Geometry: final body of the model. Coordinates: model frame, mm. A direction names the side the tool comes from. Coordinates: 2 decimals unless noted, no trailing zeros. Order: outer loops, then holes, each group sorted by start corner. A loop starts at its lowest first (then second) coordinate and runs counter-clockwise, first axis right, second up. Notation, with made-up numbers: (28.5, 34.5) -> (40.5, 34.5) arc R15 ccw to (40.5, 48.5) -> close; hole circle Ø5 at (17.25, -19.75). An arc over 180 degrees is marked (long way). Use one line per item in the form item = value.
```python
from build123d import *

# Parameters (mm, degrees)
SKETCH1_R               = 7.5
BOSS_EXTRUDE1_DEPTH     = 240
SKETCH5_R               = 8
BOSS_EXTRUDE2_DEPTH     = 20
SKETCH8_R               = 5
BOSS_EXTRUDE4_DEPTH     = 8
SKETCH9_R               = 2.5
CUT_EXTRUDE3_DEPTH      = 8
CUT_EXTRUDE3_DEPTH_BACK = 8


with BuildPart() as part:
    # Sketch1 → Boss-Extrude1 (new body)
    with BuildSketch(Plane.XY):
        Circle(SKETCH1_R)
    extrude(amount=BOSS_EXTRUDE1_DEPTH)

    # Sketch5 → Boss-Extrude2 (add)
    with BuildSketch(Plane.XY.offset(240)):
        Circle(SKETCH5_R)
    extrude(amount=BOSS_EXTRUDE2_DEPTH)

    # Sketch8 → Boss-Extrude4 (add)
    with BuildSketch(Plane(origin=(0, 0, 0), x_dir=(-1, 0, 0), z_dir=(0, 0, -1))):
        Circle(SKETCH8_R)
    extrude(amount=BOSS_EXTRUDE4_DEPTH)

    # Sketch9 → Cut-Extrude3 (cut, two sides)
    with BuildSketch(Plane(origin=(0, 0, 0), x_dir=(1, 0, 0), z_dir=(0, 1, 0))) as cut_extrude3_sk:
        with Locations((0, -250.064612311)):
            Circle(SKETCH9_R)
    extrude(amount=CUT_EXTRUDE3_DEPTH, mode=Mode.SUBTRACT)
    extrude(cut_extrude3_sk.sketch, amount=-CUT_EXTRUDE3_DEPTH_BACK, mode=Mode.SUBTRACT)


solid = part.part
```
1) Section A-A, the plane x = 0. Output: boundary loops of the cut face in (y, z), and give its area (3 significant figures).
Results found:
outline = (-8, 240) -> (-7.5, 240) -> (-7.5, 0) -> (-5, 0) -> (-5, -8) -> (5, -8) -> (5, 0) -> (7.5, 0) -> (7.5, 240) -> (8, 240) -> (8, 247.56) -> (-8, 247.56) -> close; (-8, 252.56) -> (8, 252.56) -> (8, 260) -> (-8, 260) -> close
area = 3,920 mm2
2) Section C-C, the plane z = 170.5. Output: boundary loops of the cut face in (x, y).
Results found:
outline = circle Ø15 at (0, 0)
3) Pull-direction query (Z, two-part tool) for faces 3 (the cylindrical face through (-0.542, -0.112, 252.505)), 4 (the flat face through (0, 0, -8)), 5 (the cylindrical face through (1.08, -4.88, -3.94)); classes: released by +Z, released by -Z, zero draft, split by the parting line, or undercut.
Results found:
face_3 = undercut
face_4 = released by -Z
face_5 = zero draft
4) Contact query for flat-ended pins moving along their axis: P1, Ø4, axis at x = -5, z = 123.5, coming from the -Y side; P2, Ø8, axis at x = -6, z = 91.5, coming from the +Y side; P3, Ø3, axis at y = -2, z = 43.5, coming from the +X side. Output: stop coordinate, or through.
Results found:
P1 = -6.87
P2 = 7.23
P3 = 7.48
5) Section B-B, the plane y = 0. Output: boundary loops of the cut face in (x, z).
Results found:
outline = (-8, 240) -> (-7.5, 240) -> (-7.5, 0) -> (-5, 0) -> (-5, -8) -> (5, -8) -> (5, 0) -> (7.5, 0) -> (7.5, 240) -> (8, 240) -> (8, 260) -> (-8, 260) -> close; hole circle Ø5 at (0, 250.06)
6) Access query for faces 1 (the flat face through (0, 0, 260)), 2 (the cylindrical face through (-7.493, 0.33, 118.32)). Directions: +Z, -Z, +X, -X, +Y, -Y. A direction counts if a zero-diameter tool reaches every point of the face in a straight line with its end or side. Return the directions, or none.
Results found:
face_1 = +Z, +X, -X, +Y, -Y
face_2 = -Z
7) Material intervals for probe 1 along Z at (x, y) = (0, 4.5); probe 2 along Z at (x, y) = (-0.5, -1); probe 3 along Z at (x, y) = (5.25, 1.5), sorted ascending. Write a range as from..to.
Results found:
probe_1 = -8..247.56, 252.56..260
probe_2 = -8..247.62, 252.51..260
probe_3 = 0..260
